Print and shaded views of the part. All mm, measured from the part's lowest x, y and z. A direction names the side the tool comes from. Coordinates: 2 decimals unless noted, no trailing zeros. Order: outer loops, then holes, each group sorted by start corner. A loop starts at its lowest first (then second) coordinate and runs counter-clockwise, first axis right, second up.
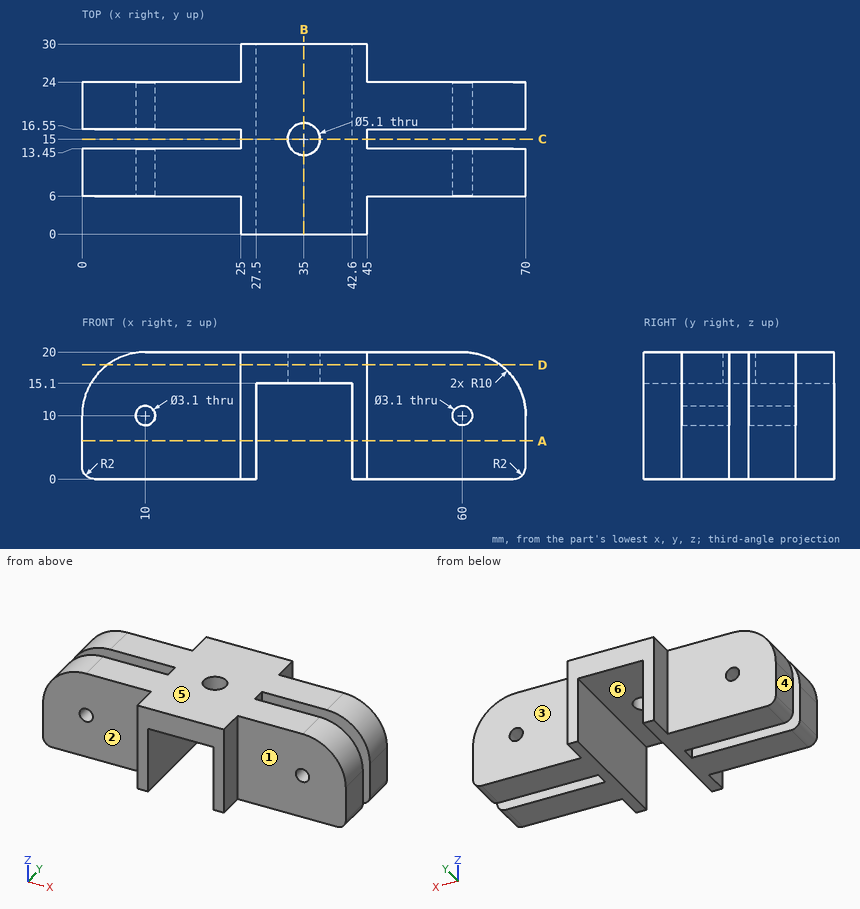
Q1. Cut at C-C, the plane y = 15. List the corners of the cut face in (x, z).
Established:
outline: (25, 0) - (27.5, 0) - (27.5, 15.1) - (32.45, 15.1) - (32.45, 20) - (25, 20) - close; (37.55, 15.1) - (42.6, 15.1) - (42.6, 0) - (45, 0) - (45, 20) - (37.55, 20) - close
Q2. Probe line 1 (Z direction, x = 10, y = 11.5); line 2 (Y direction, x = 48, z = 10.5); line 3 (Y direction, x = 35, z = 17.85). List the from-to ranges inside material, lowest first.
Established:
line 1: z = 0 to 8.45, 11.55 to 20
line 2: y = 6 to 13.45, 16.55 to 24
line 3: y = 0 to 12.45, 17.55 to 30
Q3. Cut at D-D, the plane z = 18. List the corners of the cut face in (x, y), plus the area to 3 significant figures.
Established:
outline: (4, 6) - (25, 6) - (25, 0) - (45, 0) - (45, 6) - (66, 6) - (66, 13.45) - (45, 13.45) - (45, 16.55) - (66, 16.55) - (66, 24) - (45, 24) - (45, 30) - (25, 30) - (25, 24) - (4, 24) - (4, 16.55) - (25, 16.55) - (25, 13.45) - (4, 13.45) - close; hole circle Ø5.1 at (35, 15)
area: 1,210 mm2
Q4. Which spindle directions (+Z, -Z, +X, -X, +Y, -Y) get a long thin tool onto all of the face, cutting with end or side? Do the marked faces 1, 2 and 3. Say none if no direction does.
Established:
face 1: +Z, -Z, +X, -Y
face 2: +Z, -Z, -X, -Y
face 3: +Z, -Z, +X, +Y
Q5. Drop flat-ended pins along their axis: P1, Ø10, axis at x = 62, z = 11, coming from the -Y side; P2, Ø0.9, axis at y = 15.5, z = 5.5, coming from the +X side; P3, Ø10, axis at x = 18, z = 5.5, coming from the +Y side; P4, Ø4.5, axis at x = 35, y = 15, coming from the +Z side. Give the stop position or say it passes through.
Established:
P1: stops at y = 6
P2: stops at x = 45
P3: stops at y = 24
P4: passes through
Q6. Cut at B-B, the plane x = 35. List the corners of the cut face in (y, z).
Established:
outline: (0, 15.1) - (12.45, 15.1) - (12.45, 20) - (0, 20) - close; (17.55, 15.1) - (30, 15.1) - (30, 20) - (17.55, 20) - close
Q7. Mould opens along X. For the marked faces 4, 5 and 6 say: pulls with the +X half, pulls with the -X half, needs draft (parallel to the pull), parting line crosses it, or undercut.
Established:
face 4: pulls with the -X half
face 5: needs draft
face 6: undercut
Q8. Cut at A-A, the plane z = 6. List the corners of the cut face in (x, y), plus the area to 3 significant figures.
Established:
outline: (0, 6) - (25, 6) - (25, 0) - (27.5, 0) - (27.5, 30) - (25, 30) - (25, 24) - (0, 24) - (0, 16.55) - (25, 16.55) - (25, 13.45) - (0, 13.45) - close; (42.6, 0) - (45, 0) - (45, 6) - (70, 6) - (70, 13.45) - (45, 13.45) - (45, 16.55) - (70, 16.55) - (70, 24) - (45, 24) - (45, 30) - (42.6, 30) - close
area: 892 mm2
